Check sheet for the modelled part. Datum: model origin and axes. Units: mm. A direction names the side the tool comes from. Round coordinates to 2 decimals unless told otherwise and drop trailing zeros. Write each loop counter-clockwise with the first axis right and the second up, starting at its lowest first coordinate (ties: lowest second). Pieces come first, ordered by that corner, then holes. Notation, with made-up numbers: M 17,0.25 L 28,0.25 A15 ccw 28,26.25 Z; hole C 45.5,-4.5 d1. An arc over 180 degrees is marked long. Answer in a Markdown table with one row per item.
```python
from build123d import *

# Parameters (mm, degrees)
F0_W      = 110
F0_H      = 240
F1_DEPTH  = 45
F2_W      = 105
F2_H      = 235
F3_DEPTH  = 42.5
F4_R      = 4
F5_DEPTH  = 8
F6_W      = 13
F6_H      = 13
F7_DEPTH  = 2.5
F8_W      = 7
F8_H      = 14
F9_DEPTH  = 2.5
F10_R     = 3
F11_R     = 3
F13_DEPTH = 2.5
F14_R     = 1
F23_D     = 2.5
F23_DEPTH = 10
F23_TIP   = 0.7510757738
F24_W     = 234
F24_H     = 9
F25_DEPTH = 1.4
F27_DEPTH = 234
F29_D     = 5.1
F29_DEPTH = 8
F29_TIP   = 1.5321945785
F17_W     = 15
F17_H     = 15
F30_DEPTH = 10
F32_DEPTH = 15
F34_DEPTH = 15
F35_D     = 2.5
F35_DEPTH = 10
F35_TIP   = 0.7510757738
F37_D     = 2.5
F37_DEPTH = 7
F37_TIP   = 0.7510757738


with BuildPart() as f1:
    # F0 (on Top) → F1 (new body)
    with BuildSketch(Plane.XY):
        Rectangle(F0_W, F0_H)
    extrude(amount=F1_DEPTH)

    # F2 (on face) → F3 (cut, through all)
    with BuildSketch(Plane.XY.offset(45)):
        Rectangle(F2_W, F2_H)
    extrude(amount=-F3_DEPTH, mode=Mode.SUBTRACT)

    # F4 (on face) → F5 (join)
    with BuildSketch(Plane.XY.offset(2.5)):
        with Locations((-38, 110.5)):
            Circle(F4_R)
        with Locations((38, 110.5)):
            Circle(F4_R)
        with Locations((-38, -24.5)):
            Circle(F4_R)
        with Locations((38, -24.5)):
            Circle(F4_R)
        with Locations((-40, -52.5)):
            Circle(F4_R)
        with Locations((40, -52.5)):
            Circle(F4_R)
        with Locations((-40, -110.5)):
            Circle(F4_R)
        with Locations((40, -110.5)):
            Circle(F4_R)
    extrude(amount=F5_DEPTH)

    # F6 (on face) → F7 (cut, through all)
    with BuildSketch(Plane.YZ.offset(55)):
        with Locations((0, 17.5)):
            Rectangle(F6_W, F6_H)
    extrude(amount=-F7_DEPTH, mode=Mode.SUBTRACT)

    # F8 (on face) → F9 (cut, through all)
    with BuildSketch(Plane(origin=(-55, 0, 0), x_dir=(0, -1, 0), z_dir=(-1, 0, 0))):
        with Locations((-62.5, 28)):
            Rectangle(F8_W, F8_H)
        with Locations((-45.5, 28)):
            Rectangle(F8_W, F8_H)
        with Locations((-28.5, 28)):
            Rectangle(F8_W, F8_H)
        with Locations((-11.5, 28)):
            Rectangle(F8_W, F8_H)
        with Locations((5.5, 28)):
            Rectangle(F8_W, F8_H)
        with Locations((-79.5, 28)):
            Rectangle(F8_W, F8_H)
        with Locations((-96.5, 28)):
            Rectangle(F8_W, F8_H)
    extrude(amount=-F9_DEPTH, mode=Mode.SUBTRACT)

    # F10
    f10_edges = [f1.edges().sort_by_distance(p)[0] for p in [
        (-55, -120, 22.5),
        (55, -120, 22.5),
        (-55, 120, 22.5),
        (55, 120, 22.5),
    ]]
    fillet(f10_edges, radius=F10_R)

    # F11
    f11_edges = [f1.edges().sort_by_distance(p)[0] for p in [
        (-52.5, -117.5, 23.75),
        (52.5, -117.5, 23.75),
        (-52.5, 117.5, 23.75),
        (52.5, 117.5, 23.75),
    ]]
    fillet(f11_edges, radius=F11_R)

    # F12 (on face) → F13 (cut, through all)
    with BuildSketch(Plane.YZ.offset(55)):
        with BuildLine():
            ThreePointArc((-33.9475087821, 10.5), (-26.699664275, 13.5021554928), (-23.6975087821, 20.75))
            ThreePointArc((-23.6975087821, 20.75), (-41.1953532893, 27.9978445072), (-33.9475087821, 10.5))
        make_face()
    extrude(amount=-F13_DEPTH, mode=Mode.SUBTRACT)

    # F14
    f14_edges = [f1.edges().sort_by_distance(p)[0] for p in [
        (0, -120, 45),
        (55, -33.947509, 31),
        (55, -6.5, 17.5),
        (55, 0, 11),
        (55, 6.5, 17.5),
        (55, 0, 24),
        (-55, 100, 28),
        (-55, 93, 28),
        (-55, 96.5, 21),
        (-55, 96.5, 35),
        (-55, 79.5, 35),
        (-55, 83, 28),
        (-55, 79.5, 21),
        (-55, 76, 28),
        (-55, 62.5, 35),
        (-55, 66, 28),
        (-55, 62.5, 21),
        (-55, 59, 28),
        (-55, 45.5, 35),
        (-55, 42, 28),
        (-55, 49, 28),
        (-55, 45.5, 21),
        (-55, 32, 28),
        (-55, 28.5, 21),
        (-55, 28.5, 35),
        (-55, 25, 28),
        (-55, 15, 28),
        (-55, 11.5, 21),
        (-55, 11.5, 35),
        (-55, 8, 28),
        (-55, -5.5, 35),
        (-55, -2, 28),
        (-55, -9, 28),
        (-55, -5.5, 21),
    ]]
    fillet(f14_edges, radius=F14_R)

    # F17 (on offset) → F19 section 0
    with BuildSketch(Plane.XY.offset(42.5), mode=Mode.PRIVATE) as f19_s0:
        Polygon((-52.5, 117.5), (-52.5, 102.5), (-37.5, 117.5), align=None)
    loft([f19_s0.sketch, Vertex(-52.5, 117.5, 32.5)])

    # F17 (on offset) → F20 section 0
    with BuildSketch(Plane.XY.offset(42.5), mode=Mode.PRIVATE) as f20_s0:
        Polygon((37.5, 117.5), (52.5, 102.5), (52.5, 117.5), align=None)
    loft([f20_s0.sketch, Vertex(52.5, 117.5, 32.5)])

    # F17 (on offset) → F21 section 0
    with BuildSketch(Plane.XY.offset(42.5), mode=Mode.PRIVATE) as f21_s0:
        Polygon((37.5, -117.5), (52.5, -117.5), (52.5, -102.5), align=None)
    loft([f21_s0.sketch, Vertex(52.5, -117.5, 32.5)])

    # F17 (on offset) → F22 section 0
    with BuildSketch(Plane.XY.offset(42.5), mode=Mode.PRIVATE) as f22_s0:
        Polygon((-52.5, -117.5), (-37.5, -117.5), (-52.5, -102.5), align=None)
    loft([f22_s0.sketch, Vertex(-52.5, -117.5, 32.5)])

    # F23
    with Locations(Plane.XY.offset(42.5)):
        with Locations((-47.5, -112.5), (-47.5, 112.5), (47.5, 112.5), (47.5, -112.5)):
            Hole(F23_D / 2, depth=F23_DEPTH)
            with Locations((0, 0, -(F23_DEPTH + F23_TIP / 2))):  # 118° drill point
                Cone(0, F23_D / 2, F23_TIP, mode=Mode.SUBTRACT)

    # F24 (on face) → F25 (join)
    with BuildSketch(Plane(origin=(-55, 0, 0), x_dir=(0, -1, 0), z_dir=(-1, 0, 0))):
        with Locations((0, 12.5)):
            Rectangle(F24_W, F24_H)
    extrude(amount=F25_DEPTH)

    # F26 (on face) → F27 (cut, through all)
    with BuildSketch(Plane.XZ.offset(117)):
        Polygon((-56.4, 16), (-55, 17), (-56.4, 17), align=None)
        Polygon((-56.4, 8), (-55, 8), (-56.4, 9), align=None)
    extrude(amount=-F27_DEPTH, mode=Mode.SUBTRACT)

    # F29
    with Locations(Plane(origin=(-56.4, 0, 0), x_dir=(0, -1, 0), z_dir=(-1, 0, 0))):
        with Locations((34, 12.5), (-34, 12.5), (-100, 12.5), (100, 12.5)):
            Hole(F29_D / 2, depth=F29_DEPTH)
            with Locations((0, 0, -(F29_DEPTH + F29_TIP / 2))):  # 118° drill point
                Cone(0, F29_D / 2, F29_TIP, mode=Mode.SUBTRACT)

    # F17 (on offset) → F30 (join)
    with BuildSketch(Plane.XY.offset(42.5)):
        with Locations((-45, -20)):
            Rectangle(F17_W, F17_H)
        with Locations((45, -20)):
            Rectangle(F17_W, F17_H)
    extrude(amount=-F30_DEPTH)

    # F31 (on face) → F32 (cut, through all)
    with BuildSketch(Plane.XZ.offset(27.5)):
        Polygon((-37.5, 42.5), (-52.5, 32.5), (-37.5, 32.5), align=None)
    extrude(amount=-F32_DEPTH, mode=Mode.SUBTRACT)

    # F33 (on face) → F34 (cut, through all)
    with BuildSketch(Plane.XZ.offset(27.5)):
        Polygon((52.5, 32.5), (37.5, 42.5), (37.5, 32.5), align=None)
    extrude(amount=-F34_DEPTH, mode=Mode.SUBTRACT)

    # F35
    with Locations(Plane.XY.offset(42.5)):
        with Locations((-47.5, -20), (47.5, -20)):
            Hole(F35_D / 2, depth=F35_DEPTH)
            with Locations((0, 0, -(F35_DEPTH + F35_TIP / 2))):  # 118° drill point
                Cone(0, F35_D / 2, F35_TIP, mode=Mode.SUBTRACT)

    # F37 (one way)
    with BuildSketch(Plane.XY.offset(10.5)):
        with Locations((-38, -24.5), (-40, -52.5), (40, -52.5), (38, -24.5), (-40, -110.5), (38, 110.5), (40, -110.5), (-38, 110.5)):
            Circle(F37_D / 2)
    extrude(amount=-F37_DEPTH, mode=Mode.SUBTRACT)
    with Locations(Plane.XY.offset(10.5)):
        with Locations((-38, -24.5), (-40, -52.5), (40, -52.5), (38, -24.5), (-40, -110.5), (38, 110.5), (40, -110.5), (-38, 110.5)):
            with Locations((0, 0, -(F37_DEPTH + F37_TIP / 2))):  # 118° drill point
                Cone(0, F37_D / 2, F37_TIP, mode=Mode.SUBTRACT)


solid = f1.part
```
1. Section check A-A, the plane y = 80. Record the cut outline in (x, z), and give its area (3 significant figures).
Found:
| item | result |
|---|---|
| outline | M -56.4,9 L -55,8 L -55,0 L 55,0 L 55,44 A1 ccw 54,45 L 52.5,45 L 52.5,2.5 L -52.5,2.5 L -52.5,21 L -54,21 A1 ccw -55,20 L -55,17 L -56.4,16 Z; M -55,36 A1 ccw -54,35 L -52.5,35 L -52.5,45 L -54,45 A1 ccw -55,44 Z |
| area | 463 mm2 |
2. Go/stop test with flat-tipped pins: pin 1 (1.5 mm diameter, centred on x = -32, y = -32, fed in from +Z); pin 2 (2.5 mm diameter, centred on x = -41, y = -112, fed in from +Z); pin 3 (4 mm diameter, centred on y = -1, z = 21, fed in from +X); pin 4 (16.5 mm diameter, centred on x = -42, y = 112, fed in from +Z). Record where each tip stops, or that it passes through.
Found:
| item | result |
|---|---|
| pin 1 | stops at z = 2.5 |
| pin 2 | stops at z = 10.5 |
| pin 3 | stops at x = -52.5 |
| pin 4 | stops at z = 45 |
3. Section check B-B, the plane x = 7. Record the cut outline in (y, z).
Found:
| item | result |
|---|---|
| outline | M -120,0 L 120,0 L 120,44 A1 ccw 119,45 L 117.5,45 L 117.5,2.5 L -117.5,2.5 L -117.5,45 L -119,45 A1 ccw -120,44 Z |
4. Access from +Z, -Z, +X, -X, +Y, -Y to the whole of each face (thin tool, end or side, straight path). Record for faces 1 (the face through (-54.423, -97.644, 11.523)), 2 (the face through (55, -2, 27)), 3 (the face through (-47, -27.5, 39)), 4 (the face through (-44.895, -20.105, 37.57)).
Found:
| item | result |
|---|---|
| face 1 | -X |
| face 2 | +Z, -Z, +X, +Y, -Y |
| face 3 | +Z |
| face 4 | none |
5. Scan lines: L1, parallel to X at y = 16.5, z = 36; L2, parallel to X at y = 80, z = 12; L3, parallel to Y at x = -13, z = 43. Record each from-to range of solid material in increasing order.
Found:
| item | result |
|---|---|
| L1 | x = -55 to -52.5, 52.5 to 55 |
| L2 | x = -56.4 to -52.5, 52.5 to 55 |
| L3 | y = -120 to -117.5, 117.5 to 120 |
6. Draft check along Y on faces 5 (the face through (-1, 2, 2.5)), 6 (the face through (-1, 120, 22)), 7 (the face through (-55, -1.6, 36.3)). Enter one of: +Y half, -Y half, draft (parallel to the pull), parting line (faces both ways), or undercut.
Found:
| item | result |
|---|---|
| face 5 | undercut |
| face 6 | +Y half |
| face 7 | draft |
